CAD build for the part. Positions are in the model's coordinates, mm. A direction names the side the tool comes from. Give positions to 0.01 mm unless a question says otherwise; leave off trailing zeros. Write each loop counter-clockwise with the first axis right and the second up, starting at its lowest first coordinate (ties: lowest second). Pieces come first, ordered by that corner, then holes. Notation, with made-up numbers: (29, 73) - (61, 73) arc R22 ccw to (61, 97) - close; hole circle Ø5 at (63, 40). An arc over 180 degrees is marked (long way). Answer as a JSON object with one key per item and string values.
from build123d import *

# Parameters (mm, degrees)
F0_W         = 53.0858039856
F0_H         = 43.5083806515
F1_DEPTH     = 48.3354907483
F2_W         = 29.9567952752
F2_H         = 35.2134015411
F3_DEPTH     = 53.0868039856
F11_W        = 12.8029063344
F11_H        = 17.8795624524
F12_DEPTH    = 13.5525853763
F13_R        = 6.3133849469
F4_DEPTH     = 13.5525853763
F5_SIZE      = 12.7
F14_T1_DEPTH = 107.6402324205
F6_W         = 13.5556794703
F6_H         = 17.6709126681
F15_DEPTH    = 17.3024511896
F7_W         = 6.7778397352
F7_H         = 30.6645780802
F7_W_2       = 9.8140304908
F7_H_2       = 48.3354907483
F8_DEPTH     = 43.2281381166
F9_W         = 6.7778397352
F9_H         = 13.1220892072
F10_DEPTH    = 25.925686927


# Not quite as in the source:
# - a fillet or chamfer that OpenCascade refuses, or shapes differently, is made with other operations: its cross-section is extruded or revolved along the edge and cut away or added


with BuildPart() as f1:
    # F0 (on Top) → F1 (new body)
    with BuildSketch(Plane.XY):
        Rectangle(F0_W, F0_H)
    extrude(amount=F1_DEPTH)

    # F2 (on face) → F3 (cut, through all)
    with BuildSketch(Plane.YZ.offset(26.5429019928)):
        with Locations((-6.7757926881, 30.7287899777)):
            Rectangle(F2_W, F2_H)
    extrude(amount=-F3_DEPTH, mode=Mode.SUBTRACT)

    # F11 (on face) → F12 (cut, through all)
    with BuildSketch(Plane.XZ.offset(-8.2026049495)):
        with Locations((-0.513387844, 39.3957095221)):
            Rectangle(F11_W, F11_H)
    extrude(amount=-F12_DEPTH, mode=Mode.SUBTRACT)

    # F13 (on face) → F4 (cut, through all)
    with BuildSketch(Plane.XZ.offset(-8.2026049495)):
        with Locations((-0.513387844, 30.4559282959)):
            Circle(F13_R)
    extrude(amount=-F4_DEPTH, mode=Mode.SUBTRACT)

    # F5
    f5_edges = [f1.edges().sort_by_distance(p)[0] for p in [
        (26.542902, -21.75419, 6.561045),
        (-26.542902, -21.75419, 6.561045),
    ]]
    chamfer(f5_edges, length=F5_SIZE)

    # F14: fillet of radius 45.6724150938 on 2 edges, made by hand

    # F14_s2 → F14_t1 (cut)
    with BuildSketch(Plane.XY.offset(-47.2590716067)):
        with BuildLine():
            ThreePointArc((5.0607266499, -21.7541903257), (-11.9692421066, -18.4604215607), (-26.5429019928, -9.0541903257))
            Line((-26.5429019928, -9.0541903257), (-13.8429019928, -21.7541903257))
            Line((-13.8429019928, -21.7541903257), (5.0607266499, -21.7541903257))
        make_face()
        with BuildLine():
            ThreePointArc((-5.0607266499, -21.7541903257), (11.9692421066, -18.4604215607), (26.5429019928, -9.0541903257))
            Line((26.5429019928, -9.0541903257), (13.8429019928, -21.7541903257))
            Line((13.8429019928, -21.7541903257), (-5.0607266499, -21.7541903257))
        make_face()
    extrude(amount=F14_T1_DEPTH, mode=Mode.SUBTRACT)

    # F6 (on face) → F15 (cut)
    with BuildSketch(Plane(origin=(0, 21.7541903257, 0), x_dir=(-1, 0, 0), z_dir=(0, 1, 0))):
        with Locations((-19.7650622576, 8.8354563341)):
            Rectangle(F6_W, F6_H)
    extrude(amount=-F15_DEPTH, mode=Mode.SUBTRACT)

    # F7 (on face) → F8 (cut, through all)
    with BuildSketch(Plane(origin=(0, 21.7541903257, 0), x_dir=(-1, 0, 0), z_dir=(0, 1, 0))):
        with Locations((-23.1539821252, 33.0032017082)):
            Rectangle(F7_W, F7_H)
        with Locations((21.6358867474, 24.1677453741)):
            Rectangle(F7_W_2, F7_H_2)
    extrude(amount=-F8_DEPTH, mode=Mode.SUBTRACT)

    # F9 (on face) → F10 (cut, through all)
    with BuildSketch(Plane(origin=(0, 4.4517391361, 0), x_dir=(-1, 0, 0), z_dir=(0, 1, 0))):
        with Locations((-23.1539821252, 6.5610446036)):
            Rectangle(F9_W, F9_H)
    extrude(amount=-F10_DEPTH, mode=Mode.SUBTRACT)


solid = f1.part
Item 1: Cut at B-B (z = 10). Give the cut face in (x, y).
Entries:
{"outline": "(-16.73, -16.22) arc R45.67 ccw to (0, -21.47) arc R45.67 ccw to (19.77, -14.42) - (19.77, 4.45) - (12.99, 4.45) - (12.99, 21.75) - (-16.73, 21.75) - close"}
Item 2: Which spindle directions (+Z, -Z, +X, -X, +Y, -Y) get a long thin tool onto all of the face, cutting with end or side? Do faces 4 (the flat face through (2, -7, 13.122)), 5 (the flat face through (-6.915, 15, 39)), 6 (the flat face through (12.987, 13, 9)). Say none if no direction does.
Entries:
{"face 4": "+Z, +X, -X, -Y", "face 5": "+Z, +Y, -Y", "face 6": "-Z, +X, +Y"}
Item 3: Mould opens along X. For faces 1 (the cylindrical face through (-0.652, 14.884, 24.144)), 2 (the flat face through (19.765, 15, 33)), 3 (the flat face through (13, 15, 48.335)) say: +X half, -X half, draft (parallel to the pull), parting line (faces both ways), or undercut.
Entries:
{"face 1": "undercut", "face 2": "+X half", "face 3": "draft"}
Item 4: Cut at A-A (z = 33). Give the cut face in (x, y), and give its area (3 significant figures).
Entries:
{"outline": "(-16.73, 8.2) - (-6.91, 8.2) - (-6.91, 21.75) - (-16.73, 21.75) - close; (5.89, 8.2) - (19.77, 8.2) - (19.77, 21.75) - (5.89, 21.75) - close", "area": "321 mm2"}
Item 5: Flat gauge pins, fed straight in: P1, Ø17.5, axis at x = -4, z = 35.5, coming from the -Y side; P2, Ø3.5, axis at x = 18, y = 15.5, coming from the -Z side; P3, Ø2, axis at x = 17, z = 3.5, coming from the +Y side. Where does each tip first touch, or does it go through?
Entries:
{"P1": "y = 8.2", "P2": "z = 17.67", "P3": "y = 4.45"}
Item 6: Cut at D-D (x = 16.5). Give the cut face in (y, z), and give its area (3 significant figures).
Entries:
{"outline": "(-16.34, 0) - (4.45, 0) - (4.45, 13.12) - (-16.34, 13.12) - close; (8.2, 17.67) - (21.75, 17.67) - (21.75, 48.34) - (8.2, 48.34) - close", "area": "688 mm2"}
Item 7: Cut at C-C (y = 11). Give the cut face in (x, z), and give its area (3 significant figures).
Entries:
{"outline": "(-16.73, 0) - (12.99, 0) - (12.99, 17.67) - (19.77, 17.67) - (19.77, 48.34) - (5.89, 48.34) - (5.89, 30.46) - (5.8, 30.46) arc R6.31 cw to (-6.83, 30.46) - (-6.91, 30.46) - (-6.91, 48.34) - (-16.73, 48.34) - close", "area": "1,350 mm2"}
Item 8: Probe line 1 (X direction, y = 17.5, z = 36.5); line 2 (Y direction, x = 2, z = 20); line 3 (Z direction, x = 4, y = -10). List the from-to ranges inside material, lowest first. Write a range as from..to.
Entries:
{"line 1": "-16.73..-6.91, 5.89..19.77", "line 2": "8.2..21.75", "line 3": "0..13.12"}
